Autodesk Fusion 360 part; units mm, degrees
sketch "Sketch1" plane through (0, 0, 0) normal (0, 0, 1) x (1, 0, 0)
  line L0 (0, 0) -> (104, 0)
  line L1 (104, 0) -> (104, 51)
  line L2 (104, 51) -> (0, 51)
  line L3 (0, 51) -> (0, 0)
  dimension "d1" = 104
  dimension "d2" = 51
extrude "Extrude1" add sketch "Sketch1" along normal blind 4
fillet "Fillet1" radius 2.5 4 edges at (104, 0, 2) (0, 0, 2) (104, 51, 2) (0, 51, 2)
sketch "Sketch2" plane through (0, 0, 4) normal (0, 0, 1) x (-1, 0, 0)
  arc A0 (-2.5, -51) -> (0, -48.5) centre (-2.5, -48.5) ccw
  line L0 (0, -48.5) -> (0, -2.5)
  arc A1 (0, -2.5) -> (-2.5, 0) centre (-2.5, -2.5) ccw
  line L1 (-2.5, 0) -> (-101.5, 0)
  arc A2 (-101.5, 0) -> (-104, -2.5) centre (-101.5, -2.5) ccw
  line L2 (-104, -2.5) -> (-104, -48.5)
  arc A3 (-104, -48.5) -> (-101.5, -51) centre (-101.5, -48.5) ccw
  line L3 (-101.5, -51) -> (-2.5, -51)
sketch "Sketch3" plane through (0, 0, 4) normal (0, 0, 1) x (-1, 0, 0)
  line L0 (2, -53) -> (-106, -53)
  line L1 (-106, -53) -> (-106, 2)
  line L2 (-106, 2) -> (2, 2)
  line L3 (2, 2) -> (2, -53)
  line L4 (-2.5, 0) -> (-101.5, 0)
  line L5 (-104, -2.5) -> (-104, -48.5)
  line L6 (0, -48.5) -> (0, -2.5)
  line L7 (-101.5, -51) -> (-2.5, -51)
  dimension "d7" = 2
  dimension "d8" = 2
  dimension "d9" = 2
  dimension "d10" = 2
sketch "Sketch6" plane through (0, 0, 0) normal (0, 0, 1) x (1, 0, 0)
  line L0 (-2.5, -2.5) -> (106.5, -2.5)
  line L1 (106.5, -2.5) -> (106.5, 53.5)
  line L2 (106.5, 53.5) -> (-2.5, 53.5)
  line L3 (-2.5, 53.5) -> (-2.5, -2.5)
  line L4 (2.5, 0) -> (101.5, 0)
  line L5 (104, 2.5) -> (104, 48.5)
  line L6 (101.5, 51) -> (2.5, 51)
  line L7 (0, 48.5) -> (0, 2.5)
  dimension "d15" = 2.5
  dimension "d16" = 2.5
  dimension "d17" = 2.5
  dimension "d18" = 2.5
extrude "Extrude3" add sketch "Sketch6" against normal blind 3
fillet "Fillet3" radius 2.5 4 edges at (-2.5, 53.5, -1.5) (106.5, 53.5, -1.5) (106.5, -2.5, -1.5) (-2.5, -2.5, -1.5)
sketch "Sketch7" plane through (0, 0, 4) normal (0, 0, 1) x (-1, 0, 0)
  circle A0 centre (-34, -46.5) radius 2.5
  line L0 (-104, -2.5) -> (-104, -48.5)
  line L1 (-101.5, -51) -> (-2.5, -51)
  line L2 (-36.5, -46.5) -> (-36.5, -51)
  line L3 (-31.5, -46.5) -> (-31.5, -51)
  dimension "d23" = 5
  dimension "d24" = 70
  dimension "d25" = 4.5
extrude "Extrude4" cut sketch "Sketch7" against normal blind 11
sketch "Sketch8" plane through (0, 0, -3) normal (0, 0, -1) x (1, 0, 0)
  line L0 (36.5, -51) -> (31.5, -51)
  line L1 (31.5, -51) -> (31.5, -46.5)
  arc A0 (36.5, -46.5) -> (31.5, -46.5) centre (34, -46.5) ccw
  line L2 (36.5, -46.5) -> (36.5, -51)
  arc A1 (0, 2.5) -> (-2.5, 0) centre (0, 0) ccw
  line L3 (-2.5, 0) -> (-2.5, -51)
  arc A2 (-2.5, -51) -> (0, -53.5) centre (0, -51) ccw
  line L4 (0, -53.5) -> (104, -53.5)
  arc A3 (104, -53.5) -> (106.5, -51) centre (104, -51) ccw
  line L5 (106.5, -51) -> (106.5, 0)
  arc A4 (106.5, 0) -> (104, 2.5) centre (104, 0) ccw
  line L6 (104, 2.5) -> (0, 2.5)
  line L7 (31.5, -51) -> (31.5, -53.5)
  line L8 (36.5, -51) -> (36.5, -53.5)
extrude "Extrude5" cut sketch "Sketch8" against normal blind 4 contours L0 L4 L7 L8
sketch "Sketch9" plane through (0, 0, 4) normal (0, 0, 1) x (-1, 0, 0)
sketch "Sketch10" plane through (0, 0, 4) normal (0, 0, 1) x (-1, 0, 0)
sketch "Sketch11" plane through (0, 0, -3) normal (0, 0, -1) x (1, 0, 0)
  line L0 (36.5, -46.5) -> (36.5, -53.5)
  line L1 (36.5, -53.5) -> (104, -53.5)
  arc A0 (104, -53.5) -> (106.5, -51) centre (104, -51) ccw
  line L2 (106.5, -51) -> (106.5, 0)
  arc A1 (106.5, 0) -> (104, 2.5) centre (104, 0) ccw
  line L3 (104, 2.5) -> (0, 2.5)
  arc A2 (0, 2.5) -> (-2.5, 0) centre (0, 0) ccw
  line L4 (-2.5, 0) -> (-2.5, -51)
  arc A3 (-2.5, -51) -> (0, -53.5) centre (0, -51) ccw
  line L5 (0, -53.5) -> (31.5, -53.5)
  line L6 (31.5, -53.5) -> (31.5, -46.5)
  arc A4 (36.5, -46.5) -> (31.5, -46.5) centre (34, -46.5) ccw
  line L7 (70, -53.5) -> (74, -53.5)
  line L8 (74, -53.5) -> (74, -46.5)
  line L9 (74, -46.5) -> (70, -46.5)
  line L10 (70, -46.5) -> (70, -53.5)
  circle A5 centre (72, -46.5) radius 2
  dimension "d30" = 32.5
  dimension "d31" = 4
  dimension "d32" = 7
extrude "Extrude6" cut sketch "Sketch11" against normal blind 9 contours L1 L7 L8 L10 A5 | L9 A5 | L9 A5
extrude "Extrude7" add sketch "Sketch7" against normal blind 7
extrude "Extrude8" add sketch "Sketch8" against normal blind 3 contours L0 L4 L7 L8
extrude "Extrude9" add sketch "Sketch2" along normal blind 2
extrude "Extrude10" cut 1 faces at (71.3333, 49.5, 4) along direction (0, 0, 1) blind 9
extrude "Extrude11" add 1 faces at (-2.5, 34, -1) along direction (-1, 0, 0) blind 5
fillet "Fillet4" radius 2.5 4 edges at (-7.5, 51, -1.5) (-2.5, 51, -1.5) (-2.5, 0, -1.5) (-7.5, 0, -1.5)
sketch "Sketch12" plane through (0, 0, 0) normal (0, 1, 0) x (1, 0, 0)
extrude "Extrude12" [suppressed]
extrude "Extrude2" [suppressed]
fillet "Fillet2" [suppressed]
sketch "Sketch4" plane through (0, 0, 0) normal (0, 0, 1) x (1, 0, 0)
sketch "Sketch5" plane through (0, 0, 0) normal (0, 0, 1) x (1, 0, 0)
Here's how the part is built. I have some questions about the finished solid (model axes, mm). A direction names the side the tool comes from. Coordinates: 2 decimals unless noted, no trailing zeros. Write each loop counter-clockwise with the first axis right and the second up, starting at its lowest first coordinate (ties: lowest second). Pieces come first, ordered by that corner, then holes.
1) Which directions (+Z, -Z, +X, -X, +Y, -Y) give clear straight access to the entire face, cutting with the end or side of a thin tool? Please do faces 1 (the face through (88, 51, 3)), 2 (the face through (0, 26, 3)), 3 (the face through (0.713, 50.248, 2.958)).
Filled in:
face 1: +Z, +X, -X, +Y
face 2: +Z, -X, +Y, -Y
face 3: +Z, -X, +Y
2) If I drill on line 1 (X direction, y = 48, z = 1.75); line 2 (Y direction, x = 93.5, z = 5.5); line 3 (X direction, y = 36.5, z = 1.25), over which ranges is the centre line in solid material (lowest first)?
Filled in:
line 1: x = 0 to 70, 74 to 104
line 2: y = 0 to 51
line 3: x = 0 to 104
3) If we section it at B-B (z = 1.5): List the corners of the cut face in (x, y) for me, plus the area to 3 significant figures.
Filled in:
outline: (0, 2.5) arc R2.5 ccw to (2.5, 0) - (101.5, 0) arc R2.5 ccw to (104, 2.5) - (104, 48.5) arc R2.5 ccw to (101.5, 51) - (74, 51) - (74, 46.5) arc R2 cw to (70, 46.5) - (70, 51) - (2.5, 51) arc R2.5 ccw to (0, 48.5) - close
area: 5,270 mm2
4) Thinking about a two-plate mould opening in X: for faces 4 (the face through (74, 49, 1)), 5 (the face through (35, 53.5, -2)), 6 (the face through (-7.5, 26, -1)), which applies, +X half, -X half, draft (parallel to the pull), parting line (faces both ways), or undercut?
Filled in:
face 4: undercut
face 5: draft
face 6: -X half
5) If we section it at D-D (x = 72): List the corners of the cut face in (y, z) for me, plus the area to 3 significant figures.
Filled in:
outline: (-2.5, -3) - (44.5, -3) - (44.5, 6) - (0, 6) - (0, 0) - (-2.5, 0) - close
area: 408 mm2
6) If we section it at C-C (y = 40): List the corners of the cut face in (x, z) for me, plus the area to 3 significant figures.
Filled in:
outline: (-7.5, -3) - (106.5, -3) - (106.5, 0) - (104, 0) - (104, 6) - (0, 6) - (0, 0) - (-7.5, 0) - close
area: 966 mm2
7) I'm going to push flat-ended pins straight in: pin 1 (0.7 mm diameter, centred on x = -4.5, z = -2, fed in from +Y); pin 2 (5 mm diameter, centred on x = 92, z = 4.5, fed in from -Y); pin 3 (3 mm diameter, centred on y = 20.5, z = 4.5, fed in from -X). Where does each tip first touch, or does it pass through?
Filled in:
pin 1: stops at y = 51.01
pin 2: stops at y = 0
pin 3: stops at x = 0
8) If we section it at A-A (x = 51): List the corners of the cut face in (y, z) for me.
Filled in:
outline: (-2.5, -3) - (53.5, -3) - (53.5, 0) - (51, 0) - (51, 6) - (0, 6) - (0, 0) - (-2.5, 0) - close
